```python
from build123d import *

# Parameters (mm, degrees)
SKETCH033_R             = 11
SKETCH033_R_2           = 4
PAD012_DEPTH            = 7
SKETCH035_R             = 5.6
SKETCH035_R_2           = 5.5
POCKET016_DEPTH         = 1.5
SKETCH034_R             = 5.6
SKETCH034_R_2           = 5.5
POCKET019_DEPTH         = 3
SKETCH032_R             = 9.1
SKETCH032_R_2           = 9
POCKET018_DEPTH         = 1
SKETCH031_R             = 9.1
SKETCH031_R_2           = 9
POCKET017_DEPTH         = 1
FILLET002_R             = 0.2
BODY008_PITCH_ANGLE     = -90
BODY008_PLACEMENT_ANGLE = 90


with BuildPart() as part:
    # Sketch033 → Pad012 (new body)
    with BuildSketch(Plane.XY):
        Circle(SKETCH033_R)
        Circle(SKETCH033_R_2, mode=Mode.SUBTRACT)
    extrude(amount=PAD012_DEPTH)

    # Sketch035 (on Face4 of Pad012) → Pocket016 (cut, symmetric)
    with BuildSketch(Plane.XY.offset(7)):
        Circle(SKETCH035_R)
        Circle(SKETCH035_R_2, mode=Mode.SUBTRACT)
    extrude(amount=POCKET016_DEPTH, both=True, mode=Mode.SUBTRACT)

    # Sketch034 (on Face2 of Pocket016) → Pocket019 (cut)
    with BuildSketch(Plane(origin=(0, 0, 0), x_dir=(1, 0, 0), z_dir=(0, 0, -1))):
        Circle(SKETCH034_R)
        Circle(SKETCH034_R_2, mode=Mode.SUBTRACT)
    extrude(amount=-POCKET019_DEPTH, mode=Mode.SUBTRACT)

    # Sketch032 (on Face3 of Pocket019) → Pocket018 (cut)
    with BuildSketch(Plane.XY.offset(7)):
        Circle(SKETCH032_R)
        Circle(SKETCH032_R_2, mode=Mode.SUBTRACT)
    extrude(amount=-POCKET018_DEPTH, mode=Mode.SUBTRACT)

    # Sketch031 (on Face2 of Pocket018) → Pocket017 (cut)
    with BuildSketch(Plane(origin=(0, 0, 0), x_dir=(1, 0, 0), z_dir=(0, 0, -1))):
        Circle(SKETCH031_R)
        Circle(SKETCH031_R_2, mode=Mode.SUBTRACT)
    extrude(amount=-POCKET017_DEPTH, mode=Mode.SUBTRACT)

    # Fillet002
    fillet002_edges = [part.edges().sort_by_distance(p)[0] for p in [
        (-11, 0, 0),
        (-11, 0, 7),
    ]]
    fillet(fillet002_edges, radius=FILLET002_R)


with BuildPart() as part_1:
    # Body008 pitch: moved
    add(part.part.rotate(Axis((0, 0, 0), (0, 1, 0)), BODY008_PITCH_ANGLE))


with BuildPart() as part_2:
    # Body008 placement: moved
    add(part_1.part.moved(Location((0, 94.2, 58.6))).rotate(Axis((0, 94.2, 58.6), (0, 0, 1)), BODY008_PLACEMENT_ANGLE))


solid = part_2.part
```
For this review, take the finished solid that the model builds, in its own axes (mm). Round coordinates to 2 decimals unless told otherwise and drop trailing zeros. Order: outer loops, then holes, each group sorted by start corner. A loop starts at its lowest first (then second) coordinate and runs counter-clockwise, first axis right, second up. Notation, with made-up numbers: (-31.75, 16) -> (21.25, 16) arc R33 cw to (21.25, 44) -> close; hole circle Ø2 at (35, 53). An arc over 180 degrees is marked (long way). Use a Markdown table: item, result.
Item 1: Take a section at A-A (y = 93.5). State the section outline as (x, z) points.
Resolved:
| item | result |
|---|---|
| outline | circle Ø22 at (0, 58.6); circle Ø18 at (0, 58.6); circle Ø11 at (0, 58.6); hole circle Ø18.2 at (0, 58.6); hole circle Ø11.2 at (0, 58.6); hole circle Ø8 at (0, 58.6) |
Item 2: Take a section at C-C (y = 89.5). State the section outline as (x, z) points, plus the area to 3 significant figures.
Resolved:
| item | result |
|---|---|
| outline | circle Ø22 at (0, 58.6); hole circle Ø8 at (0, 58.6) |
| area | 330 mm² |
Item 3: Draft analysis for pull direction X (two halves, no side actions). For faces 1 (the flat face through (4, 87.2, 54)), 2 (the cylindrical face through (4.213, 90.746, 68.761)), 3 (the cylindrical face through (-0.176, 90.749, 54.604)), state which applies: +X half, -X half, draft (parallel to the pull), parting line (faces both ways), or undercut.
Resolved:
| item | result |
|---|---|
| face 1 | draft |
| face 2 | parting line |
| face 3 | undercut |
Item 4: Take a section at B-B (y = 91.5). State the section outline as (x, z) points, plus the area to 3 significant figures.
Resolved:
| item | result |
|---|---|
| outline | circle Ø22 at (0, 58.6); circle Ø11 at (0, 58.6); hole circle Ø11.2 at (0, 58.6); hole circle Ø8 at (0, 58.6) |
| area | 326 mm² |
Item 5: For line 1 along X through (y, z) = (90, 58.6); line 2 along X through (y, z) = (93.75, 65.75); line 3 along Z through (x, y) = (-8, 88), list the stretches that pass through material, from the lowest coordinate up. Write a range as [from, to].
Resolved:
| item | result |
|---|---|
| line 1 | x = [-11, -4], [4, 11] |
| line 2 | x = [-8.36, -5.63], [-5.47, 5.47], [5.63, 8.36] |
| line 3 | z = [51.05, 54.26], [54.48, 62.72], [62.94, 66.15] |
